from build123d import *

# Parameters (mm, degrees)
SKETCH4_R          = 5.8166
SKETCH4_R_2        = 5.65785
CUT_EXTRUDE2_DEPTH = 7.112
CUT_EXTRUDE1_DEPTH = 7.112
CIRPATTERN1_COUNT  = 18


with BuildPart() as part:
    # Sketch1 → Revolve1 (revolve)
    with BuildSketch(Plane.XY, mode=Mode.PRIVATE) as revolve1_sk:
        with BuildLine():
            Line((-8.7376, 2.38125), (8.7376, 2.38125))
            Line((8.7376, 2.38125), (8.7376, 8.001))
            Line((8.7376, 8.001), (7.7343, 8.001))
            ThreePointArc((7.7343, 8.001), (7.002290733, 7.337844347), (6.731, 6.3881))
            Line((6.731, 6.3881), (6.731, 5.8166))
            Line((6.731, 5.8166), (-0.381, 5.8166))
            Line((-0.381, 5.8166), (-0.381, 6.3881))
            ThreePointArc((-0.381, 6.3881), (-0.652290733, 7.337844347), (-1.3843, 8.001))
            Line((-1.3843, 8.001), (-2.3876, 8.001))
            Line((-2.3876, 8.001), (-2.3876, 6.35))
            Line((-2.3876, 6.35), (-8.7376, 6.35))
            Line((-8.7376, 6.35), (-8.7376, 2.38125))
        make_face()
    revolve(revolve1_sk.sketch.rotate(Axis((-8.7376, 0, 0), (1, 0, 0)), 90), axis=Axis((-8.7376, 0, 0), (1, 0, 0)))

    # Sketch4 → Cut-Extrude2 (cut)
    with BuildSketch(Plane(origin=(-0.381, 0, 0), x_dir=(0, 0, -1), z_dir=(1, 0, 0))):
        Circle(SKETCH4_R)
        Circle(SKETCH4_R_2, mode=Mode.SUBTRACT)
    extrude(amount=CUT_EXTRUDE2_DEPTH, mode=Mode.SUBTRACT)

    # Sketch3 → Cut-Extrude1 (cut)
    with BuildSketch(Plane(origin=(-0.381, 0, 0), x_dir=(0, 0, -1), z_dir=(1, 0, 0))):
        with BuildLine():
            Line((-0.64235315, 5.621267566), (-0.342998874, 4.97930025))
            Line((-0.342998874, 4.97930025), (0.342998874, 4.97930025))
            Line((0.342998874, 4.97930025), (0.64235315, 5.621267566))
            ThreePointArc((0.64235315, 5.621267566), (0, 5.65785), (-0.64235315, 5.621267566))
        make_face()
    cut_extrude1 = extrude(amount=CUT_EXTRUDE1_DEPTH, mode=Mode.SUBTRACT)

    # CirPattern1: Cut-Extrude1 ×18 about axis
    cirpattern1_axis = Axis((0, 0, 0), (1, 0, 0))
    for i in range(1, CIRPATTERN1_COUNT):
        add(cut_extrude1.rotate(cirpattern1_axis, i * 360 / CIRPATTERN1_COUNT), mode=Mode.SUBTRACT)


solid = part.part
Verification items for the finished model (mm, model axes). A direction names the side the tool comes from. Round coordinates to 2 decimals unless told otherwise and drop trailing zeros. Loops run counter-clockwise (first coordinate to the right, second up) from the corner with the lowest first, then second, coordinate; pieces in that order, holes last. Notation, with made-up numbers: (56, 23) - (66, 23) arc R11 cw to (66, 28) - close; hole circle Ø4 at (14.5, 47.5). An arc over 180 degrees is marked (long way). Answer in a Markdown table with one row per item. Add a question column.
Q1. Section check A-A on z = 0. Enter the section's corners in (x, y).
Q2. Gauge pin test, flat ends, axial feed: pin 1 (6 mm diameter, centred on x = -6, z = 5.5, fed in from -Y); pin 2 (1 mm diameter, centred on x = 4.5, y = 2.5, fed in from +Z); pin 3 (2 mm diameter, centred on x = -3, z = -2.5, fed in from -Y). Record the tip position at first contact, or that the pin passes through.
Q3. Section check D-D on x = 7.5. Enter the section's corners in (y, z), plus the area to 3 significant figures.
Q4. Section check B-B on y = 0. Enter the section's corners in (x, z), plus the area to 3 significant figures.
Q5. Section check C-C on x = -6.75. Enter the section's corners in (y, z).
Q6. Tool access check on faces 1 (the face through (-1.89, 7.81, -1.73)), 2 (the face through (-0.381, 5, -2)), 3 (the face through (-5.61, 3.86, -5.04)). Record the directions out of +Z, -Z, +X, -X, +Y, -Y that give a thin tool (end or side, any length) a straight path to the whole face; none if there is none.
Q7. Material ranges on line 1 (Y direction, x = 0.25, z = 0); line 2 (Y direction, x = 5.5, z = 4.25); line 3 (Y direction, x = -3.5, z = 1.25), recorded low to high.
Q8. Release check for a two-part mould opening along X. For faces 4 (the face through (6.731, 5, 2)), 5 (the face through (8.23, 7.81, -1.73)), 6 (the face through (-8.738, 0, 3)) record: pulls with the +X half, pulls with the -X half, needs draft (parallel to the pull), parting line crosses it, or undercut.
Found:
| question | item | result |
|---|---|---|
| 1 | outline | (-8.74, -6.35) - (-2.39, -6.35) - (-2.39, -8) - (-1.38, -8) arc R1.8 ccw to (-0.38, -6.39) - (-0.38, -4.98) - (6.73, -4.98) - (6.73, -6.39) arc R1.8 ccw to (7.73, -8) - (8.74, -8) - (8.74, -2.38) - (-8.74, -2.38) - close; (-8.74, 2.38) - (8.74, 2.38) - (8.74, 8) - (7.73, 8) arc R1.8 ccw to (6.73, 6.39) - (6.73, 4.98) - (-0.38, 4.98) - (-0.38, 6.39) arc R1.8 ccw to (-1.38, 8) - (-2.39, 8) - (-2.39, 6.35) - (-8.74, 6.35) - close |
| 2 | pin 1 | stops at y = -5.84 |
| 2 | pin 2 | stops at z = 5.29 |
| 2 | pin 3 | stops at y = -7.82 |
| 3 | outline | circle Ø15.73 at (0, 0); hole circle Ø4.76 at (0, 0) |
| 3 | area | 176 mm² |
| 4 | outline | (-8.74, -6.35) - (-2.39, -6.35) - (-2.39, -8) - (-1.38, -8) arc R1.8 ccw to (-0.38, -6.39) - (-0.38, -5.66) - (6.73, -5.66) - (6.73, -6.39) arc R1.8 ccw to (7.73, -8) - (8.74, -8) - (8.74, -2.38) - (-8.74, -2.38) - close; (-8.74, 2.38) - (8.74, 2.38) - (8.74, 8) - (7.73, 8) arc R1.8 ccw to (6.73, 6.39) - (6.73, 5.66) - (-0.38, 5.66) - (-0.38, 6.39) arc R1.8 ccw to (-1.38, 8) - (-2.39, 8) - (-2.39, 6.35) - (-8.74, 6.35) - close |
| 4 | area | 140 mm² |
| 5 | outline | circle Ø12.7 at (0, 0); hole circle Ø4.76 at (0, 0) |
| 6 | face 1 | +X, -X |
| 6 | face 2 | none |
| 6 | face 3 | -X |
| 7 | line 1 | y = -4.98 to -2.38, 2.38 to 4.98 |
| 7 | line 2 | y = -3.73 to -2.94, -2.6 to 2.6, 2.94 to 3.73 |
| 7 | line 3 | y = -6.23 to -2.03, 2.03 to 6.23 |
| 8 | face 4 | undercut |
| 8 | face 5 | needs draft |
| 8 | face 6 | pulls with the -X half |
